Verification items for the finished model (mm, model axes). Face numbers are marked on the shaded views. Give positions to 0.01 mm unless a question says otherwise; leave off trailing zeros. Write each loop counter-clockwise with the first axis right and the second up, starting at its lowest first coordinate (ties: lowest second). Pieces come first, ordered by that corner, then holes. Notation, with made-up numbers: (21, 57) -> (65, 57) arc R19 ccw to (65, 88) -> close; hole circle Ø5 at (-25, -16.5). An arc over 180 degrees is marked (long way). Write item = value, one per line.
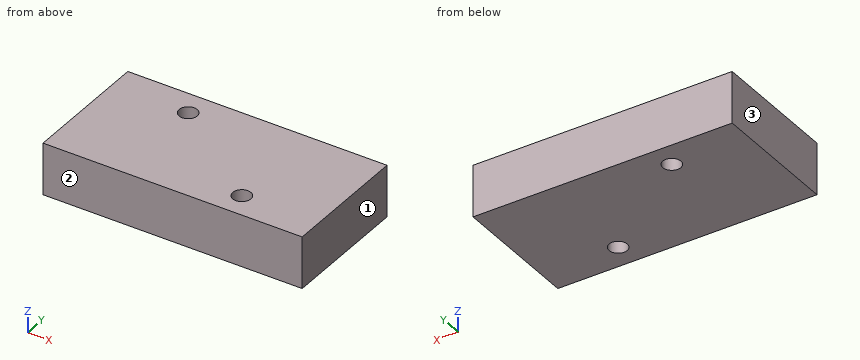
from build123d import *

# Parameters (mm, degrees)
SKETCH1_W           = 50
SKETCH1_H           = 25
BOSS_EXTRUDE1_DEPTH = 10
SKETCH2_R           = 1.75
CUT_EXTRUDE1_DEPTH  = 10
SKETCH3_R           = 1.75
CUT_EXTRUDE2_DEPTH  = 10


with BuildPart() as part:
    # Sketch1 → Boss-Extrude1 (new body)
    with BuildSketch(Plane.XY):
        with Locations((-6.627906977, 5.813953488)):
            Rectangle(SKETCH1_W, SKETCH1_H)
    extrude(amount=BOSS_EXTRUDE1_DEPTH)

    # Sketch2 → Cut-Extrude1 (cut)
    with BuildSketch(Plane.XY.offset(10)):
        with Locations((-16.877906977, 13.563953488)):
            Circle(SKETCH2_R)
    extrude(amount=-CUT_EXTRUDE1_DEPTH, mode=Mode.SUBTRACT)

    # Sketch3 → Cut-Extrude2 (cut)
    with BuildSketch(Plane.XY.offset(10)):
        with Locations((3.622093023, -1.936046512)):
            Circle(SKETCH3_R)
    extrude(amount=-CUT_EXTRUDE2_DEPTH, mode=Mode.SUBTRACT)


solid = part.part
Item 1: Sectioned sample at C-C on z = 6.5. Record the cut outline in (x, y).
Response values:
outline = (-31.63, -6.69) -> (18.37, -6.69) -> (18.37, 18.31) -> (-31.63, 18.31) -> close; hole circle Ø3.5 at (-16.88, 13.56); hole circle Ø3.5 at (3.62, -1.94)
Item 2: Sectioned sample at A-A on y = -2.75. Record the cut outline in (x, z).
Response values:
outline = (-31.63, 0) -> (2.07, 0) -> (2.07, 10) -> (-31.63, 10) -> close; (5.17, 0) -> (18.37, 0) -> (18.37, 10) -> (5.17, 10) -> close
Item 3: Sectioned sample at B-B on x = 2.5. Record the cut outline in (y, z), then the cut area to 3 significant figures.
Response values:
outline = (-6.69, 0) -> (-3.28, 0) -> (-3.28, 10) -> (-6.69, 10) -> close; (-0.59, 0) -> (18.31, 0) -> (18.31, 10) -> (-0.59, 10) -> close
area = 223 mm^2
Item 4: Mould release check, pull along X, two halves, no side actions. Record for the marked faces 1, 2 and 3: +X half, -X half, draft (parallel to the pull), parting line (faces both ways), or undercut.
Response values:
face_1 = +X half
face_2 = draft
face_3 = -X half
Item 5: Material ranges on line 1 (X direction, y = -1.75, z = 3.25); line 2 (X direction, y = 13.25, z = 6.75); line 3 (Y direction, x = 4, z = 2.75), recorded low to high.
Response values:
line_1 = -31.63 to 1.88, 5.36 to 18.37
line_2 = -31.63 to -18.6, -15.16 to 18.37
line_3 = -6.69 to -3.64, -0.23 to 18.31
